from build123d import *

# Parameters (mm, degrees)
SKETCH_1_R      = 1
EXTRUDE_1_DEPTH = 4
FILLET_1_R      = 2
FILLET_2_R      = 1


with BuildPart() as part:
    # 草图1 → 凸台-拉伸1 (new body)
    with BuildSketch(Plane(origin=(0, 0, 0), x_dir=(1, 0, 0), z_dir=(0, 1, 0))):
        with BuildLine():
            Line((15, 20), (25, 30))
            Line((25, 30), (25, 40))
            Line((25, 40), (30, 45))
            Line((30, 45), (30, 65))
            Line((30, 65), (36, 65))
            Line((36, 65), (36, 43.100505063))
            Line((36, 43.100505063), (30.563454525, 37.663959588))
            Line((30.563454525, 37.663959588), (30.563454525, 25.663959588))
            Line((30.563454525, 25.663959588), (19.956852807, 15.05735787))
            ThreePointArc((19.956852807, 15.05735787), (17.652275132, 17.7030275), (15, 20))
        make_face()
        with Locations(Location((33, 60, 0), (0, 0, 270))):
            Circle(SKETCH_1_R, mode=Mode.SUBTRACT)
        with Locations(Location((33, 52, 0), (0, 0, 270))):
            Circle(SKETCH_1_R, mode=Mode.SUBTRACT)
    extrude(amount=EXTRUDE_1_DEPTH)

    # 圆角1
    fillet_1_edges = [part.edges().sort_by_distance(p)[0] for p in [
        (30, 2, -45),
        (30, 2, -65),
        (36, 2, -65),
        (36, 2, -43.100505063),
        (30.563454525, 2, -37.663959588),
        (30.563454525, 2, -25.663959588),
        (25, 2, -30),
    ]]
    fillet(fillet_1_edges, radius=FILLET_1_R)

    # 圆角2
    fillet_2_edges = [part.edges().sort_by_distance(p)[0] for p in [
        (19.956852807, 2, -15.05735787),
    ]]
    fillet(fillet_2_edges, radius=FILLET_2_R)


solid = part.part
Verification items for the finished model (mm, model axes). A direction names the side the tool comes from. Round coordinates to 2 decimals unless told otherwise and drop trailing zeros. Loops run counter-clockwise (first coordinate to the right, second up) from the corner with the lowest first, then second, coordinate; pieces in that order, holes last. Notation, with made-up numbers: (72, 64.25) - (117, 64.25) arc R14 ccw to (117, 78.25) - close; hole circle Ø3 at (35, 83.25). An arc over 180 degrees is marked (long way). Use a Markdown table: item, result. Add a question column.
1. Access from +Z, -Z, +X, -X, +Y, -Y to the whole of each face (thin tool, end or side, straight path). Record for faces 1 (the face through (30.563, 2, -32)), 2 (the face through (30, 2, -54)), 3 (the face through (28, 4, -39)).
2. Release check for a two-part mould opening along Z. For faces 4 (the face through (20, 2, -25)), 5 (the face through (35.84, 2.03, -43.15)), 6 (the face through (33.676, 1.972, -60.737)) record: released by +Z, released by -Z, zero draft, split by the parting line, or undercut.
3. Gauge pin test, flat ends, axial feed: pin 1 (10 mm diameter, centred on x = 19, z = -32, fed in from -Y); pin 2 (2 mm diameter, centred on y = 2, z = -36.5, fed in from -X); pin 3 (1.2 mm diameter, centred on y = 1.5, z = -30, fed in from +X). Record the tip position at first contact, or that the pin passes through.
4. Thickness scan on probe 1 along X at (y, z) = (2.3, -52); probe 2 along X at (y, z) = (1.15, -49); probe 3 along X at (y, z) = (3.65, -35). Record the ranges inside material, lowest first. Write a range as [from, to].
5. Section check D-D, the plane z = -54. Record the boundary of the cut face in (x, y).
6. Section check C-C, the plane y = 0.5. Record the boundary of the cut face in (x, z), plus the area to 3 significant figures.
7. Section check B-B, the plane x = 33. Record the boundary of the cut face in (y, z), plus the area to 3 significant figures.
8. Section check A-A, the plane z = -60. Record the boundary of the cut face in (x, y), plus the area to 3 significant figures.
Checks:
| question | item | result |
|---|---|---|
| 1 | face 1 | +Z, +X, +Y, -Y |
| 1 | face 2 | -Z, -X, +Y, -Y |
| 1 | face 3 | +Z, -Z, +X, -X, +Y |
| 2 | face 4 | released by -Z |
| 2 | face 5 | released by +Z |
| 2 | face 6 | undercut |
| 3 | pin 1 | passes through |
| 3 | pin 2 | stops at x = 25 |
| 3 | pin 3 | stops at x = 30.56 |
| 4 | probe 1 | x = [30, 32], [34, 36] |
| 4 | probe 2 | x = [30, 36] |
| 4 | probe 3 | x = [25, 30.56] |
| 5 | outline | (30, 0) - (36, 0) - (36, 4) - (30, 4) - close |
| 6 | outline | (15, -20) - (24.41, -29.41) arc R2 cw to (25, -30.83) - (25, -40) - (29.41, -44.41) arc R2 cw to (30, -45.83) - (30, -63) arc R2 ccw to (32, -65) - (34, -65) arc R2 ccw to (36, -63) - (36, -43.93) arc R2 ccw to (35.41, -42.51) - (31.15, -38.25) arc R2 cw to (30.56, -36.84) - (30.56, -26.49) arc R2 ccw to (29.98, -25.08) - (20.75, -15.85) arc R1 ccw to (19.27, -15.92) arc R25 cw to start; hole circle Ø2 at (33, -60); hole circle Ø2 at (33, -52) |
| 6 | area | 321 mm^2 |
| 7 | outline | (0, -65) - (4, -65) - (4, -61) - (0, -61) - close; (0, -59) - (4, -59) - (4, -53) - (0, -53) - close; (0, -51) - (4, -51) - (4, -40.1) - (0, -40.1) - close |
| 7 | area | 83.6 mm^2 |
| 8 | outline | (30, 0) - (32, 0) - (32, 4) - (30, 4) - close; (34, 0) - (36, 0) - (36, 4) - (34, 4) - close |
| 8 | area | 16.0 mm^2 |
